Source: CAD feature listing. Evaluate the final solid. Frame: model axes, mm. A direction names the side the tool comes from. Coordinates: 2 decimals unless noted, no trailing zeros. Loops run counter-clockwise (first coordinate to the right, second up) from the corner with the lowest first, then second, coordinate; pieces in that order, holes last.
Item 1: Pull-direction query (Y, two-part tool) for faces 4 (the cylindrical face through (20.826, 6.261, -0.078)), 5 (the flat face through (-19, -6.35, 0)), 6 (the flat face through (-4.448, 30, 0)); classes: +Y half, -Y half, draft (parallel to the pull), parting line (faces both ways), or undercut.
Item 2: Section query C-C, the plane z = 2.5. Return the cut outline in (x, y).
Item 3: Line query: probe 1 along X at (y, z) = (-2.5, -0.5); probe 2 along X at (y, z) = (10, -0.25); probe 3 along Y at (x, z) = (1, -1.5). Output: solid intervals per line, ascending.
Item 4: Section query A-A, the plane z = 0. Return the cut outline in (x, y) (3 decimals), then the cut area to 3 significant figures.
Item 5: Reachability of faces 1 (the flat face through (19, -6.35, 0)), 2 (the flat face through (-20.4, 0, -1.4)), 3 (the flat face through (0, 30.48, 0)) from +Z, -Z, +X, -X, +Y, -Y: full face, straight path, thin tool, end or side. Return the list, or none.
Item 6: Section query B-B, the plane y = 9.5. Return the cut outline in (x, z).
Item 7: Pin query (flat end, axial travel): pin 1 Ø0.8 at (x, z) = (2, 0.5) entering from -Y; pin 2 Ø0.6 at (x, y) = (2.5, 30) entering from +Z; pin 3 Ø1 at (x, y) = (-15.5, 20.5) entering from -Z; pin 4 Ø1.5 at (y, z) = (20.5, -1) entering from -X. Return the tip coordinate at first contact, or that it passes through.
```python
from build123d import *

# Parameters (mm, degrees)
SKETCH3_R           = 1.778
SKETCH4_R           = 3.175
BOSS_EXTRUDE1_DEPTH = 6.35
SKETCH5_R           = 3.175
BOSS_EXTRUDE2_DEPTH = 6.35
SKETCH6_W           = 8.89531995
SKETCH6_H           = 2.585925644
CUT_EXTRUDE1_DEPTH  = 2.54


with BuildPart() as part:
    # Sweep1: sweep along a path in Sketch2
    with BuildLine(Plane.XY) as sweep1_path:
        Line((-19.05, 0), (-19.05, 12.7))
        ThreePointArc((-19.05, 12.7), (0, 31.75), (19.05, 12.7))
        Line((19.05, 12.7), (19.05, 0))
    # Sketch3 → Sweep1 (sweep)
    with BuildSketch(Plane(origin=(0, 0, 0), x_dir=(1, 0, 0), z_dir=(0, 1, 0))):
        with Locations((-19.05, 0)):
            Circle(SKETCH3_R)
    sweep(path=sweep1_path.line)

    # Sketch4 → Boss-Extrude1 (add)
    with BuildSketch(Plane.XZ):
        with Locations(Location((-19.05, 0, 0), (0, 0, 270))):
            Circle(SKETCH4_R)
    extrude(amount=BOSS_EXTRUDE1_DEPTH)

    # Sketch5 → Boss-Extrude2 (add)
    with BuildSketch(Plane.XZ):
        with Locations(Location((19.05, 0, 0), (0, 0, 270))):
            Circle(SKETCH5_R)
    extrude(amount=BOSS_EXTRUDE2_DEPTH)

    # Sketch6 → Cut-Extrude1 (cut)
    with BuildSketch(Plane(origin=(0, 27.94, 0), x_dir=(1, 0, 0), z_dir=(0, 1, 0))):
        Rectangle(SKETCH6_W, SKETCH6_H)
    extrude(amount=CUT_EXTRUDE1_DEPTH, mode=Mode.SUBTRACT)


solid = part.part
```
Verdict:
1. face 4: undercut
1. face 5: -Y half
1. face 6: draft
2. outline: (-21.01, -6.35) - (-17.09, -6.35) - (-17.09, 0) - (-21.01, 0) - close; (17.09, -6.35) - (21.01, -6.35) - (21.01, 0) - (17.09, 0) - close
3. probe 1: x = -22.19 to -15.91, 15.91 to 22.19
3. probe 2: x = -20.81 to -17.29, 17.29 to 20.81
3. probe 3: y = 30.77 to 32.68
4. outline: (-22.225, -6.35) - (-15.875, -6.35) - (-15.875, 0) - (-17.272, 0) - (-17.272, 12.7) arc R17.272 cw to (-4.448, 29.39) - (-4.448, 30.48) - (4.448, 30.48) - (4.448, 29.39) arc R17.272 cw to (17.272, 12.7) - (17.272, 0) - (15.875, 0) - (15.875, -6.35) - (22.225, -6.35) - (22.225, 0) - (20.828, 0) - (20.828, 12.7) arc R20.828 ccw to (-20.828, 12.7) - (-20.828, 0) - (-22.225, 0) - close
4. area: 378 mm2
5. face 1: +Z, -Z, +X, -X, -Y
5. face 2: none
5. face 3: -Y
6. outline: circle Ø3.56 at (-19.05, 0); circle Ø3.56 at (19.05, 0)
7. pin 1: stops at y = 30.48
7. pin 2: passes through
7. pin 3: stops at z = -1.31
7. pin 4: stops at x = -19.45
